Job drawing, mm, ordinate dimensions from the low corner. One solid piece. A direction names the side the tool comes from. Round coordinates to 2 decimals unless told otherwise and drop trailing zeros. Write each loop counter-clockwise with the first axis right and the second up, starting at its lowest first coordinate (ties: lowest second). Pieces come first, ordered by that corner, then holes. Notation, with made-up numbers: (44, 27.25) - (98, 27.25) arc R10 cw to (98, 43.25) - close; hole circle Ø6 at (81.25, -1.75). An arc over 180 degrees is marked (long way). Write each question's results on one line, items separated by ' | '.
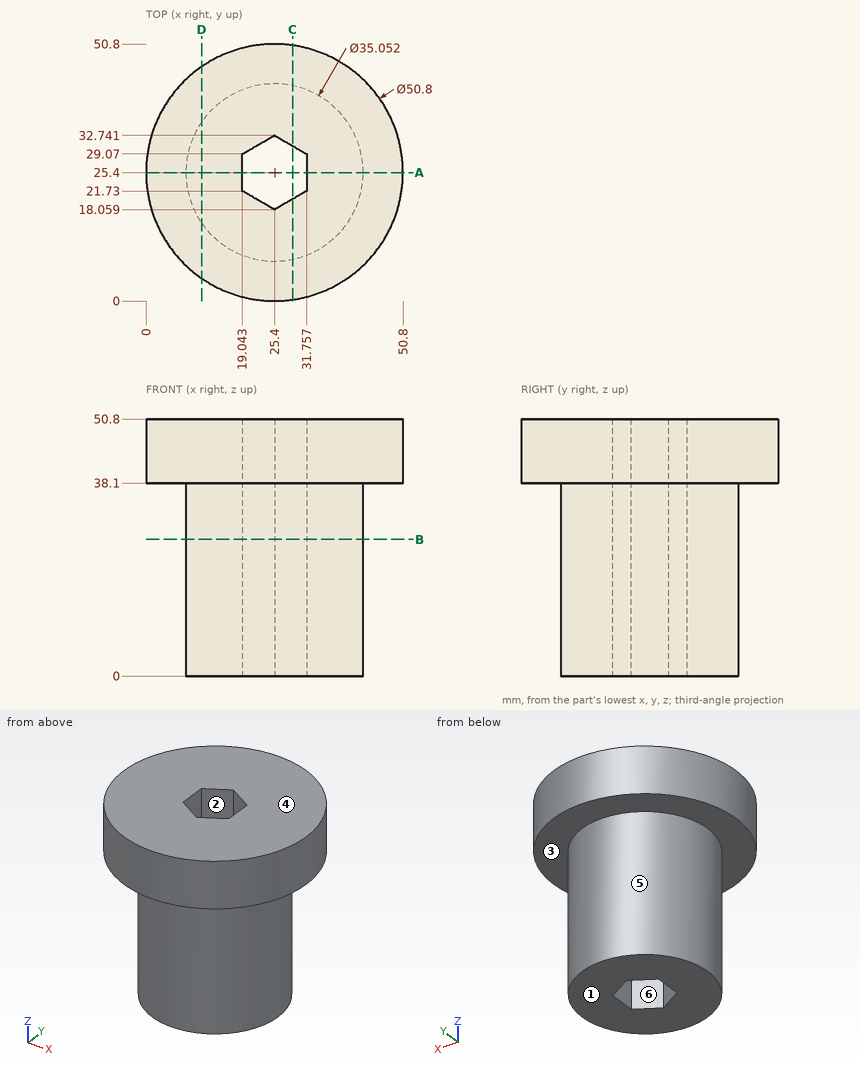
(1) Slice it at B-B, the plane z = 27. Write the cut outline in (x, y).
Worked answers:
outline: circle Ø35.05 at (25.4, 25.4); hole (19.04, 21.73) - (25.4, 18.06) - (31.76, 21.73) - (31.76, 29.07) - (25.4, 32.74) - (19.04, 29.07) - close
(2) Two-plate mould, pull along Y, no slides. Class the marked faces 4, 5 and 6: released by +Y, released by -Y, zero draft, split by the parting line, or undercut.
Worked answers:
face 4: zero draft | face 5: split by the parting line | face 6: undercut
(3) Drill centre lines: probe 1 along Z at (x, y) = (47.5, 35.5); probe 2 along Y at (x, z) = (27.5, 28.5); probe 3 along X at (y, z) = (23, 7.5). Where is each one in solid material? Low to high. Write a range as [from, to].
Worked answers:
probe 1: z = [38.1, 50.8] | probe 2: y = [8, 19.27], [31.53, 42.8] | probe 3: x = [8.04, 19.04], [31.76, 42.76]
(4) Slice it at D-D, the plane x = 11. Write the cut outline in (y, z).
Worked answers:
outline: (4.48, 38.1) - (15.41, 38.1) - (15.41, 0) - (35.39, 0) - (35.39, 38.1) - (46.32, 38.1) - (46.32, 50.8) - (4.48, 50.8) - close
(5) Slice it at A-A, the plane y = 25.4. Write the cut outline in (x, z).
Worked answers:
outline: (0, 38.1) - (7.87, 38.1) - (7.87, 0) - (19.04, 0) - (19.04, 50.8) - (0, 50.8) - close; (31.76, 0) - (42.93, 0) - (42.93, 38.1) - (50.8, 38.1) - (50.8, 50.8) - (31.76, 50.8) - close
(6) Slice it at C-C, the plane x = 29. Write the cut outline in (y, z).
Worked answers:
outline: (0.26, 38.1) - (8.25, 38.1) - (8.25, 0) - (20.14, 0) - (20.14, 50.8) - (0.26, 50.8) - close; (30.66, 0) - (42.55, 0) - (42.55, 38.1) - (50.54, 38.1) - (50.54, 50.8) - (30.66, 50.8) - close
(7) Tool access for the marked faces 1, 2 and 3: list every direction of +Z, -Z, +X, -X, +Y, -Y with a clear straight run to the whole face (end or side of a thin tool).
Worked answers:
face 1: -Z, +X, -X, +Y, -Y | face 2: +Z, -Z | face 3: -Z
(8) Flat gauge pins, fed straight in: pin 1 Ø12 at (x, z) = (20.5, 12) entering from -Y; pin 2 Ø5 at (x, z) = (20.5, 7) entering from +Y; pin 3 Ø3.5 at (y, z) = (24, 28.5) entering from -X. Where does each tip first touch, or does it go through?
Worked answers:
pin 1: stops at y = 7.87 | pin 2: stops at y = 42.76 | pin 3: stops at x = 7.87
